Source: CAD feature listing. Evaluate the final solid. Frame: model axes, mm. A direction names the side the tool comes from. Coordinates: 2 decimals unless noted, no trailing zeros. Write each loop counter-clockwise with the first axis right and the second up, starting at its lowest first coordinate (ties: lowest second). Pieces come first, ordered by that corner, then holes. Notation, with made-up numbers: M 89,19.5 L 101,19.5 A18 ccw 101,33.5 Z; hole C -0.75,-37.5 d5. An arc over 180 degrees is marked long. One line per item, written item: value. Start each with the question number.
Item 1: Cut plane C-C, the plane y = -5.75. Output: boundary loops of the cut face in (x, z).
Item 2: Set-up query: faces 4 (the cylindrical face through (-1.113, -6.261, -1.451)), 5 (the flat face through (-1.13, 3.505, 1.13)), 6 (the flat face through (-1.389, 2, 0)). Return all of +Z, -Z, +X, -X, +Y, -Y with unobstructed straight access to the full face (end or side cutting, diameter ignored); none if empty.
Item 3: Pin query (flat end, axial travel): P1, Ø2, axis at y = -3.5, z = 2, coming from the +X side; P2, Ø1, axis at y = -9, z = 1, coming from the -X side; P3, Ø1.5, axis at x = 0.5, y = -8, coming from the +Z side. Return the tip coordinate at first contact, or that it passes through.
Item 4: Mould query, pull axis Z, two halves, no side actions, for faces 1 (the flat face through (1.389, 2, 0)), 2 (the flat face through (0, -12.7, 0)), 3 (the cylindrical face through (2.846, 1.603, -0.374)). Classes: released by +Z, released by -Z, zero draft, split by the parting line, or undercut.
Item 5: Cut plane B-B, the plane z = 0. Output: boundary loops of the cut face in (x, y), then the cut area to 3 significant figures.
Item 6: Ray query, L1, parallel to X at y = 1.25, z = -0.1; L2, parallel to Y at x = 0.65, z = 0.15; L3, parallel to Y at x = -1.1, z = 1.9. Return the intervals inside material, ascending. Write a range as from..to.
Item 7: Cut plane A-A, the plane y = 2.25. Output: boundary loops of the cut face in (x, z), then the cut area to 3 significant figures.
```python
from build123d import *

# Parameters (mm, degrees)
SKETCH1_R           = 1.8288
BOSS_EXTRUDE1_DEPTH = 12.7
SKETCH2_R           = 2.8702
BOSS_EXTRUDE2_DEPTH = 3.5052
FILLET1_R           = 0.254
CUT_EXTRUDE1_DEPTH  = 2.54


with BuildPart() as part:
    # Sketch1 → Boss-Extrude1 (new body)
    with BuildSketch(Plane(origin=(0, 0, 0), x_dir=(1, 0, 0), z_dir=(0, 1, 0))):
        with Locations(Location((0, 0, 0), (0, 0, 270))):
            Circle(SKETCH1_R)
    extrude(amount=-BOSS_EXTRUDE1_DEPTH)

    # Sketch2 → Boss-Extrude2 (add)
    with BuildSketch(Plane(origin=(0, 0, 0), x_dir=(1, 0, 0), z_dir=(0, 1, 0))):
        with Locations(Location((0, 0, 0), (0, 0, 270))):
            Circle(SKETCH2_R)
    extrude(amount=BOSS_EXTRUDE2_DEPTH)

    # Fillet1
    fillet1_edges = [part.edges().sort_by_distance(p)[0] for p in [
        (0, 3.5052, -2.8702),
    ]]
    fillet(fillet1_edges, radius=FILLET1_R)

    # Sketch3 → Cut-Extrude1 (cut)
    with BuildSketch(Plane(origin=(0, 3.5052, 0), x_dir=(1, 0, 0), z_dir=(0, 1, 0))):
        Polygon((0, 1.603951217), (-1.3890625, 0.801975608), (-1.3890625, -0.801975608), (0, -1.603951217), (1.3890625, -0.801975608), (1.3890625, 0.801975608), align=None)
    extrude(amount=-CUT_EXTRUDE1_DEPTH, mode=Mode.SUBTRACT)


solid = part.part
```
From the geometry:
1. outline: C 0,0 d3.66
2. face 4: -Y
2. face 5: +Z, -Z, +X, -X, +Y
2. face 6: +Y
3. P1: stops at x = 1.53
3. P2: stops at x = -1.76
3. P3: stops at z = 1.83
4. face 1: undercut
4. face 2: zero draft
4. face 3: split by the parting line
5. outline: M -2.87,0 L -1.83,0 L -1.83,-12.7 L 1.83,-12.7 L 1.83,0 L 2.87,0 L 2.87,3.25 A0.25 ccw 2.62,3.51 L 1.39,3.51 L 1.39,0.97 L -1.39,0.97 L -1.39,3.51 L -2.62,3.51 A0.25 ccw -2.87,3.25 Z
5. area: 59.5 mm²
6. L1: x = -2.87..-1.39, 1.39..2.87
6. L2: y = -12.7..0.97
6. L3: y = 0..3.51
7. outline: C 0,0 d5.74; hole M -1.39,-0.8 L 0,-1.6 L 1.39,-0.8 L 1.39,0.8 L 0,1.6 L -1.39,0.8 Z
7. area: 19.2 mm²
